Here's how the part is built. I have some questions about the finished solid (model axes, mm). Face numbers are marked on the shaded views. A direction names the side the tool comes from. Give positions to 0.01 mm unless a question says otherwise; leave off trailing zeros. Order: outer loops, then holes, each group sorted by start corner. A loop starts at its lowest first (then second) coordinate and runs counter-clockwise, first axis right, second up.
from build123d import *

# Parameters (mm, degrees)
SKETCH1_R                    = 3.2639
BASE_FLANGE1_DEPTH           = 1.51892
EDGE_FLANGE1_STRIP_CUT_DEPTH = 15.875
EDGE_FLANGE1_DEPTH           = 15.875


# Sheet-metal steps are written as plain solids
with BuildPart() as part:
    # Sketch1 → Base-Flange1 (new body)
    with BuildSketch(Plane(origin=(0, 0, 0), x_dir=(1, 0, 0), z_dir=(0, 1, 0))):
        with BuildLine():
            Line((0, 0), (44.45, 0))
            ThreePointArc((44.45, 0), (52.3875, 7.9375), (44.45, 15.875))
            Line((44.45, 15.875), (0, 15.875))
            Line((0, 15.875), (0, 0))
        make_face()
        with Locations(Location((44.45, 7.9375, 0), (0, 0, 270))):
            Circle(SKETCH1_R, mode=Mode.SUBTRACT)
        with Locations(Location((6.35, 7.9375, 0), (0, 0, 270))):
            Circle(SKETCH1_R, mode=Mode.SUBTRACT)
    extrude(amount=-BASE_FLANGE1_DEPTH)

    # Edge-Flange1 strip (across the edge) → Edge-Flange1 strip cut (cut)
    with BuildSketch(Plane(origin=(0, -1.51892, 0), x_dir=(0.7313537016191672, -0.6819983600625019, 0), z_dir=(0, 0, -1))):
        Polygon((-7.660036486, 5.066238556), (-0.430107825, -1.675778992), (0.605793124, -0.564911227), (-6.624135537, 6.177106321), align=None)
    extrude(amount=EDGE_FLANGE1_STRIP_CUT_DEPTH, mode=Mode.SUBTRACT)

    # Edge-Flange1 section (across the edge) → Edge-Flange1 (add)
    with BuildSketch(Plane(origin=(0, -1.51892, 0), x_dir=(0.7313537016191672, -0.6819983600625019, 0), z_dir=(0, 0, -1))):
        with BuildLine():
            Line((-1.51892, 0.828317574), (-1.51892, 15.087554787))
            Line((-1.51892, 15.087554787), (0, 15.087554787))
            Line((0, 15.087554787), (0, 0.828317574))
            ThreePointArc((0, 0.828317574), (0.158000558, 0.068700598), (0.605793124, -0.564911227))
            Line((0.605793124, -0.564911227), (-0.430107825, -1.675778992))
            ThreePointArc((-0.430107825, -1.675778992), (-1.23494033, -0.536967338), (-1.51892, 0.828317574))
        make_face()
    extrude(amount=EDGE_FLANGE1_DEPTH)


solid = part.part
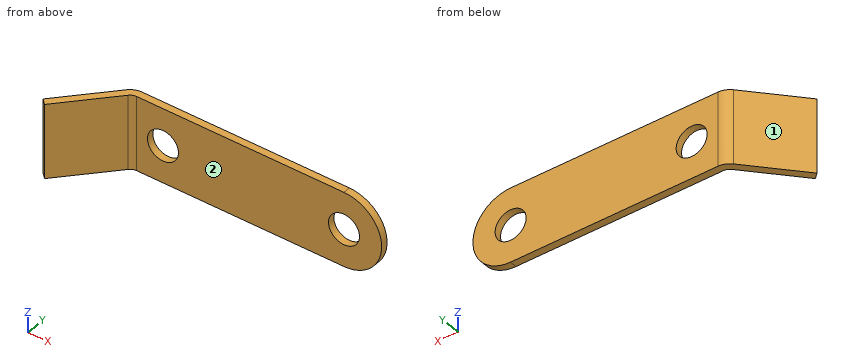
Q1. I'm going to push flat-ended pins straight in: P1, Ø8, axis at x = 38, z = -4.5, coming from the -Y side; P2, Ø1.5, axis at y = -7, z = -6.5, coming from the +X side. Where does each tip first touch, or does it pass through?
Filled sheet:
P1: stops at y = -1.52
P2: stops at x = -4.41
Q2. For the marked faces 1 and 2, which set-ups out of +Z, -Z, +X, -X, +Y, -Y let a thin tool reach every point of the face, with its end or its side?
Filled sheet:
face 1: +Z, -Z, -X, +Y
face 2: +Z, -Z, +X, -Y
Q3. I need wall thicknesses on L1, parallel to Y at x = 43, z = -11.75; L2, parallel to X at y = -1, z = -10.5; L3, parallel to X at y = -10.5, z = -10 (3 decimals). Which ranges of each line are inside material? Lowest first, please.
Filled sheet:
L1: y = -1.52 to 0
L2: x = -1.59 to 4.33, 8.37 to 42.43, 46.47 to 51.96
L3: x = -10.452 to -8.375
Q4. If we section it at D-D on x = 37.5: List the corners of the cut face in (y, z) for me (3 decimals).
Filled sheet:
outline: (-1.519, -15.875) - (0, -15.875) - (0, 0) - (-1.519, 0) - close
Q5. If we section it at C-C on z = -14.25: List the corners of the cut face in (x, y) for me (3 decimals).
Filled sheet:
outline: (-11.401, -11.517) - (-10.29, -12.553) - (-0.565, -2.125) arc R1.905 cw to (0.828, -1.519) - (49.262, -1.519) - (49.262, 0) - (0.828, 0) arc R3.424 ccw to (-1.676, -1.089) - close
Q6. If we section it at B-B on z = -7.25: List the corners of the cut face in (x, y) for me (3 decimals).
Filled sheet:
outline: (-11.401, -11.517) - (-10.29, -12.553) - (-0.565, -2.125) arc R1.905 cw to (0.828, -1.519) - (3.159, -1.519) - (3.159, 0) - (0.828, 0) arc R3.424 ccw to (-1.676, -1.089) - close; (9.541, -1.519) - (41.259, -1.519) - (41.259, 0) - (9.541, 0) - close; (47.641, -1.519) - (52.358, -1.519) - (52.358, 0) - (47.641, 0) - close
Q7. If we section it at A-A on x = 6.35: List the corners of the cut face in (y, z) for me (3 decimals).
Filled sheet:
outline: (-1.519, -15.875) - (0, -15.875) - (0, -11.201) - (-1.519, -11.201) - close; (-1.519, -4.674) - (0, -4.674) - (0, 0) - (-1.519, 0) - close
